Build history of the part. All positions in model axes, mm. Face numbers are marked on the shaded views. A direction names the side the tool comes from. Coordinates: 2 decimals unless noted, no trailing zeros. Loops run counter-clockwise (first coordinate to the right, second up) from the corner with the lowest first, then second, coordinate; pieces in that order, holes last.
Item 1: 3-axis set-ups, long thin cutter, end or side, ignore diameter. For the marked faces 1 and 2: which of +Z, -Z, +X, -X, +Y, -Y reach the whole face in a straight line?
Item 2: Cut at B-B (z = 18). List the corners of the cut face in (x, y).
Item 3: Flat gauge pins, fed straight in: pin 1 (9.5 mm diameter, centred on x = 62, z = 28, fed in from +Y); pin 2 (1.6 mm diameter, centred on x = 32.5, y = -2, fed in from -Z); pin 3 (10 mm diameter, centred on x = 12.5, z = 18, fed in from -Y); pin 4 (6 mm diameter, centred on x = 37, z = 27, fed in from -Y). Where does each tip first touch, or does it go through?
Item 4: Cut at A-A (x = 12.5). List the corners of the cut face in (y, z).
Item 5: Cut at C-C (y = 0). List the corners of the cut face in (x, z).
Item 6: Drill centre lines: line 1 along X through (y, z) = (-2, 6); line 2 along Y through (x, z) = (88, 0); line 3 along X through (y, z) = (-2.5, 26). Where is each one in solid material? Low to high.
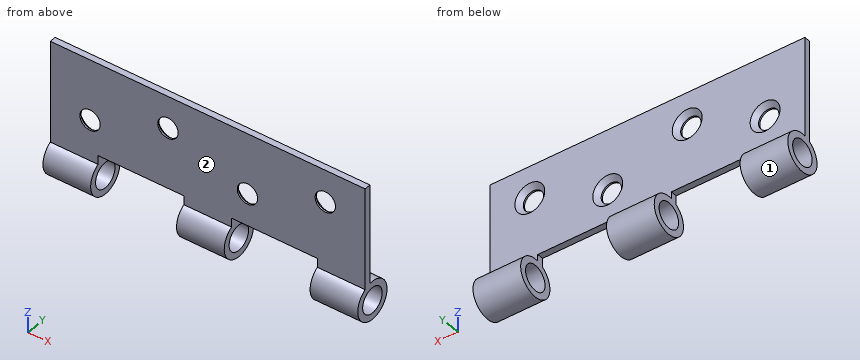
from build123d import *

# Parameters (mm, degrees)
SKETCH_1_R               = 6
SKETCH_1_R_2             = 4
EXTRUDE_1_DEPTH          = 99
SKETCH_2_W               = 99
SKETCH_2_H               = 2
EXTRUDE_2_DEPTH          = 37
SKETCH_3_R               = 4
CUT_EXTRUDE_1_DEPTH      = 106.858395983
CUT_EXTRUDE_2_DEPTH      = 106.919780967
CUT_EXTRUDE_2_DEPTH_BACK = 106.919780967
SKETCH_4_W               = 27
SKETCH_4_H               = 14
SKETCH_7_R               = 3.2
CUT_EXTRUDE_8_DEPTH      = 37
CHAMFER_1_SIZE           = 1.5


with BuildPart() as part:
    # 草图1 → 凸台-拉伸1 (new body)
    with BuildSketch(Plane(origin=(0, 0, 0), x_dir=(0, 0, -1), z_dir=(1, 0, 0))):
        Circle(SKETCH_1_R)
        Circle(SKETCH_1_R_2, mode=Mode.SUBTRACT)
    extrude(amount=EXTRUDE_1_DEPTH)

    # 草图2 → 凸台-拉伸2 (add)
    with BuildSketch(Plane.XY):
        with Locations((49.5, -2)):
            Rectangle(SKETCH_2_W, SKETCH_2_H)
    extrude(amount=EXTRUDE_2_DEPTH)

    # 草图3 → 切除-拉伸1 (cut, through all)
    with BuildSketch(Plane.ZY):
        with Locations(Location((0, 0, 0), (0, 0, 180))):
            Circle(SKETCH_3_R)
    extrude(amount=-CUT_EXTRUDE_1_DEPTH, mode=Mode.SUBTRACT)

    # 草图4 → 切除-拉伸2 (cut, two sides: drawn at the far end of the back side and taken through both)
    with BuildSketch(Plane(origin=(0, -1, 0), x_dir=(1, 0, 0), z_dir=(0, 1, 0)).offset(-CUT_EXTRUDE_2_DEPTH_BACK)):
        with Locations((28.5, -1)):
            Rectangle(SKETCH_4_W, SKETCH_4_H)
        with Locations((70.5, -1)):
            Rectangle(SKETCH_4_W, SKETCH_4_H)
    extrude(amount=CUT_EXTRUDE_2_DEPTH + CUT_EXTRUDE_2_DEPTH_BACK, mode=Mode.SUBTRACT)

    # 草图7 → 切除-拉伸8 (cut)
    with BuildSketch(Plane.XZ.offset(3)):
        with Locations((12.5, 18)):
            Circle(SKETCH_7_R)
        with Locations((37, 27)):
            Circle(SKETCH_7_R)
        with Locations((62, 18)):
            Circle(SKETCH_7_R)
        with Locations((86.5, 27)):
            Circle(SKETCH_7_R)
    extrude(amount=-CUT_EXTRUDE_8_DEPTH, mode=Mode.SUBTRACT)

    # 倒角1
    chamfer_1_edges = [part.edges().sort_by_distance(p)[0] for p in [
        (9.3, -1, 18),
        (33.8, -1, 27),
        (58.8, -1, 18),
        (83.3, -1, 27),
    ]]
    chamfer(chamfer_1_edges, length=CHAMFER_1_SIZE)


solid = part.part
Filled sheet:
1. face 1: +X, -X
1. face 2: +Z, +X, -X, -Y
2. outline: (0, -3) - (9.3, -3) - (9.3, -2.5) - (7.8, -1) - (0, -1) - close; (15.7, -3) - (58.8, -3) - (58.8, -2.5) - (57.3, -1) - (17.2, -1) - (15.7, -2.5) - close; (65.2, -3) - (99, -3) - (99, -1) - (66.7, -1) - (65.2, -2.5) - close
3. pin 1: stops at y = -1
3. pin 2: stops at z = 8
3. pin 3: stops at y = -3
3. pin 4: passes through
4. outline: (-3, 5.2) arc R6 ccw (long way) to (-1, 5.92) - (-1, 13.3) - (-2.5, 14.8) - (-3, 14.8) - close; (-3, 21.2) - (-2.5, 21.2) - (-1, 22.7) - (-1, 37) - (-3, 37) - close; hole circle Ø8 at (0, 0)
5. outline: (0, -6) - (15, -6) - (15, -4) - (0, -4) - close; (0, 4) - (15, 4) - (15, 6) - (0, 6) - close; (42, -6) - (57, -6) - (57, -4) - (42, -4) - close; (42, 4) - (57, 4) - (57, 6) - (42, 6) - close; (84, -6) - (99, -6) - (99, -4) - (84, -4) - close; (84, 4) - (99, 4) - (99, 6) - (84, 6) - close
6. line 1: x = 0 to 15, 42 to 57, 84 to 99
6. line 2: y = -6 to -4, 4 to 6
6. line 3: x = 0 to 33.96, 40.04 to 83.46, 89.54 to 99
